Could you check a few things on this model? Use its own coordinates, in mm. A direction names the side the tool comes from. Coordinates: 2 decimals unless noted, no trailing zeros. Order: outer loops, then holes, each group sorted by start corner. A loop starts at its lowest first (then second) coordinate and runs counter-clockwise, first axis right, second up. Notation, with made-up numbers: (32.5, 3) -> (45.5, 3) arc R13 cw to (45.5, 13) -> close; hole circle Ø9 at (26, -34.75). An arc over 180 degrees is marked (long way). Return JSON: item names as keys, results as strings. Group by question number.
from build123d import *

# Parameters (mm, degrees)
BOSS_EXTRUDE1_DEPTH = 4.7625
SKETCH2_R           = 3.048
CUT_EXTRUDE1_DEPTH  = 3.556
SKETCH3_R           = 1.778
CUT_EXTRUDE2_DEPTH  = 277.706047268
SKETCH4_R           = 3.048
CUT_EXTRUDE3_DEPTH  = 3.556
SKETCH5_R           = 3.048
CUT_EXTRUDE4_DEPTH  = 3.556
SKETCH6_R           = 3.048
CUT_EXTRUDE5_DEPTH  = 3.556
SKETCH7_R           = 3.048
CUT_EXTRUDE6_DEPTH  = 3.556
SKETCH8_R           = 1.778
CUT_EXTRUDE7_DEPTH  = 273.722762612
SKETCH9_R           = 1.778
CUT_EXTRUDE8_DEPTH  = 274.775889667
SKETCH10_R          = 1.778
CUT_EXTRUDE9_DEPTH  = 276.233622552
SKETCH11_R          = 1.778
CUT_EXTRUDE10_DEPTH = 276.83087619


# Read off the part's stored shape, not the designer's step: Mirror1
with BuildPart() as part:
    # Sketch1 → Boss-Extrude1 (new, symmetric)
    with BuildSketch(Plane(origin=(0, 0, 4.097149242), x_dir=(-1, 0, 0), z_dir=(0, 0, -1))):
        Polygon((-249.537325585, -63.059731366), (-240.052189426, -62.189204494), (-240.748610926, -54.601095566), (-250.233747084, -55.471622439), align=None)
        Polygon((-250.233747084, -55.471622439), (-249.537325585, -63.059731366), (-256.417466381, -63.773158253), (-256.780990146, -60.000079995), (-271.511576408, -61.370646542), (-271.864542794, -57.577031547), align=None)
        Polygon((-188.860077886, -50.394516158), (-188.325818753, -57.995763897), (-240.052189426, -62.189204494), (-240.748610926, -54.601095566), align=None)
        Polygon((-188.325818753, -57.995763897), (-178.824259081, -57.327939981), (-179.358518215, -49.726692243), (-188.860077886, -50.394516158), align=None)
        Polygon((-125.492633629, -46.578303782), (-125.059593338, -54.185989113), (-178.824259081, -57.327939981), (-179.358518215, -49.726692243), align=None)
        Polygon((-115.549986674, -53.64468875), (-115.983026964, -46.037003418), (-125.492633629, -46.578303782), (-125.059593338, -54.185989113), align=None)
        Polygon((-62.816371972, -44.102817558), (-62.616240336, -51.720188977), (-115.549986674, -53.64468875), (-115.983026964, -46.037003418), align=None)
        Polygon((-62.616240336, -51.720188977), (-53.094526063, -51.470024432), (-53.294657701, -43.852653014), (-62.816371972, -44.102817558), align=None)
        Polygon((0.217698252, -43.033956836), (0.250661746, -50.653885537), (-53.094526063, -51.470024432), (-53.294657701, -43.852653014), align=None)
        Polygon((0.250661746, -50.653885537), (5.013117184, -50.633283353), (4.98015369, -43.013354652), (0.217698252, -43.033956836), align=None)
    extrude(amount=BOSS_EXTRUDE1_DEPTH, both=True)

    # Sketch2 → Cut-Extrude1 (cut)
    with BuildSketch(Plane(origin=(-3.654807803, -39.822262509, 0), x_dir=(0.995814819891653, -0.09139389741199735, 0), z_dir=(-0.09139389741199735, -0.995814819891653, 0))):
        with Locations((249.493741553, 4.097149242)):
            Circle(SKETCH2_R)
    extrude(amount=-CUT_EXTRUDE1_DEPTH, mode=Mode.SUBTRACT)

    # Sketch3 → Cut-Extrude2 (cut, through all)
    with BuildSketch(Plane(origin=(-3.329811104, -36.28114501, 0), x_dir=(0.995814819891653, -0.09139389741199735, 0), z_dir=(-0.09139389741199735, -0.995814819891653, 0))):
        with Locations((249.493741553, 4.097149242)):
            Circle(SKETCH3_R)
    extrude(amount=-CUT_EXTRUDE2_DEPTH, mode=Mode.SUBTRACT)

    # Sketch4 → Cut-Extrude3 (cut)
    with BuildSketch(Plane(origin=(-3.130464047, -44.539122171, 0), x_dir=(0.9975390732743608, -0.07011274699317857, 0), z_dir=(-0.07011274699317857, -0.9975390732743608, 0))):
        with Locations((187.166105034, 4.097149242)):
            Circle(SKETCH4_R)
    extrude(amount=-CUT_EXTRUDE3_DEPTH, mode=Mode.SUBTRACT)

    # Sketch5 → Cut-Extrude4 (cut)
    with BuildSketch(Plane(origin=(-2.670492031, -46.915410629, 0), x_dir=(-0.998383901802788, 0.05682943445997907, 0), z_dir=(-0.05682943445997907, -0.9983839018027881, 0))):
        with Locations(Location((-123.174343872, -4.097149242, 0), (0, 0, 180))):
            Circle(SKETCH5_R)
    extrude(amount=-CUT_EXTRUDE4_DEPTH, mode=Mode.SUBTRACT)

    # Sketch6 → Cut-Extrude5 (cut)
    with BuildSketch(Plane(origin=(-1.314717641, -50.040527253, 0), x_dir=(0.9996550418058789, -0.02626399421425536, 0), z_dir=(-0.02626399421425536, -0.9996550418058789, 0))):
        with Locations((59.190519095, 4.097149242)):
            Circle(SKETCH6_R)
    extrude(amount=-CUT_EXTRUDE5_DEPTH, mode=Mode.SUBTRACT)

    # Sketch7 → Cut-Extrude6 (cut)
    with BuildSketch(Plane(origin=(-0.219127188, -50.654021954, 0), x_dir=(-0.9999906431736124, 0.004325917847692405, 0), z_dir=(-0.004325917847692405, -0.9999906431736125, 0))):
        with Locations((4.794034853, -4.097149242)):
            Circle(SKETCH7_R)
    extrude(amount=-CUT_EXTRUDE6_DEPTH, mode=Mode.SUBTRACT)

    # Sketch8 → Cut-Extrude7 (cut, through all)
    with BuildSketch(Plane(origin=(-0.203744224, -47.098055227, 0), x_dir=(0.9999906431736124, -0.004325917847692406, 0), z_dir=(-0.004325917847692406, -0.9999906431736125, 0))):
        with Locations((-4.794034853, 4.097149242)):
            Circle(SKETCH8_R)
    extrude(amount=-CUT_EXTRUDE7_DEPTH, mode=Mode.SUBTRACT)

    # Sketch9 → Cut-Extrude8 (cut, through all)
    with BuildSketch(Plane(origin=(-1.221322877, -46.485753925, 0), x_dir=(0.9996550418058789, -0.02626399421425536, 0), z_dir=(-0.02626399421425536, -0.9996550418058789, 0))):
        with Locations((59.190519095, 4.097149242)):
            Circle(SKETCH9_R)
    extrude(amount=-CUT_EXTRUDE8_DEPTH, mode=Mode.SUBTRACT)

    # Sketch10 → Cut-Extrude9 (cut, through all)
    with BuildSketch(Plane(origin=(-2.468406562, -43.365157475, 0), x_dir=(0.998383901802788, -0.05682943445997909, 0), z_dir=(-0.05682943445997909, -0.9983839018027881, 0))):
        with Locations((123.174343872, 4.097149242)):
            Circle(SKETCH10_R)
    extrude(amount=-CUT_EXTRUDE9_DEPTH, mode=Mode.SUBTRACT)

    # Sketch11 → Cut-Extrude10 (cut, through all)
    with BuildSketch(Plane(origin=(-2.881143118, -40.991873227, 0), x_dir=(-0.9975390732743608, 0.07011274699317857, 0), z_dir=(-0.07011274699317857, -0.9975390732743608, 0))):
        with Locations(Location((-187.166105034, -4.097149242, 0), (0, 0, 180))):
            Circle(SKETCH11_R)
    extrude(amount=-CUT_EXTRUDE10_DEPTH, mode=Mode.SUBTRACT)

    # Mirror1: part across plane


with BuildPart() as part_1:
    add(part.part)
    add(part.part.mirror(Plane(origin=(-4.793989996, 0.020738601, 8.859649242), x_dir=(0, 0, 1), z_dir=(-0.9999906431736159, 0.004325917846891031, 0))))


solid = part_1.part
Q1. I want a section at A-A on x = -112. Please give me the cut outline in (y, z).
Q2. I'm going to push flat-ended pins straight in: pin 1 Ø4 at (x, z) = (22, 4) entering from +Y; pin 2 Ø2 at (x, z) = (59, 2) entering from -Y. Where does each tip first touch, or does it pass through?
Q3. I want a section at B-B on x = 204. Please give me the cut outline in (y, z), and give its area (3 significant figures).
Q4. I need wall thicknesses on line 1 along Y through (x, z) = (55, 8); line 2 along Y through (x, z) = (124.5, 4.5). Which ranges of each line are inside material? Lowest first, please. Write a range as from..to.
Q5. On a 3-axis mill with a long thin cutter (end or side, diameter ignored), from which of +Z, -Z, +X, -X, +Y, -Y can I reach the whole of each face in a straight line? I mean faces 1 (the flat face through (152.803, -48.175, 4.03)), 2 (the flat face through (-223.93, -58.17, 4.03)). Say none if no direction works.
Response values:
{
 "1": {"outline": "(-52.22, -0.67) -> (-44.6, -0.67) -> (-44.6, 8.86) -> (-52.22, 8.86) -> close"},
 "2": {"pin 1": "stops at y = -43.34", "pin 2": "stops at y = -51.65"},
 "3": {"outline": "(-59.27, -0.67) -> (-51.62, -0.67) -> (-51.62, 8.86) -> (-59.27, 8.86) -> close", "area": "72.8 mm²"},
 "4": {"line 1": "y = -51.52..-43.9", "line 2": "y = -54.15..-46.52"},
 "5": {"face 1": "+Z, -Z, +X, +Y", "face 2": "+Z, -Z, -Y"}
}
